Verification items for this drawing (mm, ordinates from the low corner). Round coordinates to 2 decimals unless told otherwise and drop trailing zeros. Loops run counter-clockwise (first coordinate to the right, second up) from the corner with the lowest first, then second, coordinate; pieces in that order, holes last. Notation, with made-up numbers: (46.5, 82.25) -> (95.5, 82.25) arc R31 cw to (95.5, 120.25) -> close; hole circle Ø1 at (64, 72.5). An arc over 180 degrees is marked (long way). One line per item, written item: value. Start each with the question number.
1. Go/stop test with flat-tipped pins: pin 1 (2 mm diameter, centred on x = 206, z = 65, fed in from +Y); pin 2 (12 mm diameter, centred on x = 366, z = 100, fed in from +Y). Record where each tip stops, or that it passes through.
2. Cross-section at B-B on z = 253. Record the cut outline in (x, y) (3 decimals).
3. Material ranges on L1, parallel to Y at x = 41, z = 108; L2, parallel to Y at x = 229.5, z = 253, recorded low to high.
4. Cross-section at C-C on z = 118. Record the cut outline in (x, y) (3 decimals).
5. Cross-section at A-A on x = 275. Record the cut outline in (y, z) (3 decimals).
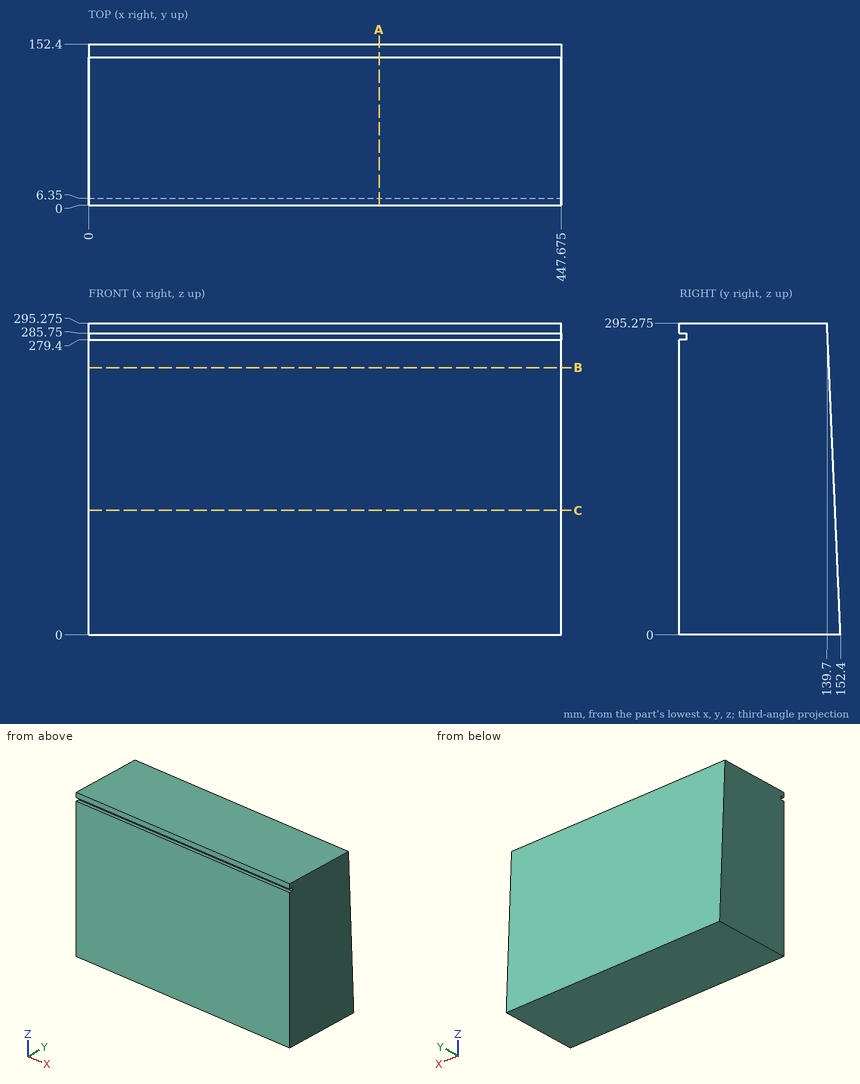
Taken from the geometry:
1. pin 1: stops at y = 149.65
1. pin 2: stops at y = 148.36
2. outline: (0, 0) -> (447.675, 0) -> (447.675, 141.518) -> (0, 141.518) -> close
3. L1: y = 0 to 147.75
3. L2: y = 0 to 141.52
4. outline: (0, 0) -> (447.675, 0) -> (447.675, 147.325) -> (0, 147.325) -> close
5. outline: (0, 0) -> (152.4, 0) -> (139.7, 295.275) -> (0, 295.275) -> (0, 285.75) -> (6.35, 285.75) -> (6.35, 279.4) -> (0, 279.4) -> close
